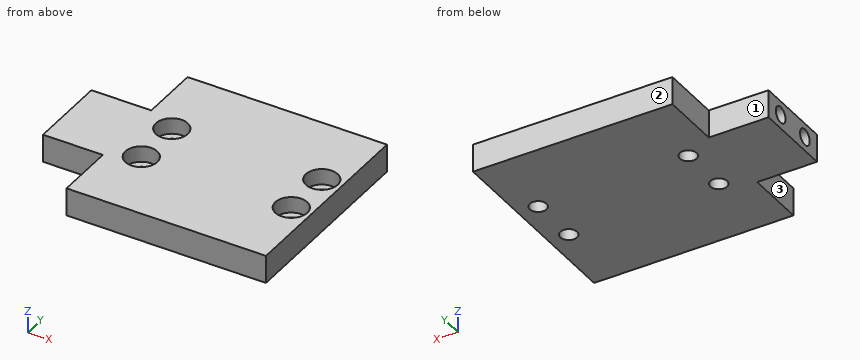
```python
from build123d import *

# Parameters (mm, degrees)
F1_DEPTH       = 7
F3_D           = 4
F3_DEPTH       = 6
F3_TIP         = 1.2017212381
F5_D           = 4.2
F5_CBORE_D     = 8
F5_CBORE_DEPTH = 4


with BuildPart() as f1:
    # F0 (on Top) → F1 (new body)
    with BuildSketch(Plane.XY):
        Polygon((32.5, -25), (32.5, 25), (-17.5, 25), (-17.5, 10), (-32.5, 10), (-32.5, -10), (-17.5, -10), (-17.5, -25), align=None)
    extrude(amount=F1_DEPTH)

    # F3
    with Locations(Plane(origin=(-32.5, 0, 0), x_dir=(0, -1, 0), z_dir=(-1, 0, 0))):
        with Locations((-5, 3.5), (5, 3.5)):
            Hole(F3_D / 2, depth=F3_DEPTH)
            with Locations((0, 0, -(F3_DEPTH + F3_TIP / 2))):  # 118° drill point
                Cone(0, F3_D / 2, F3_TIP, mode=Mode.SUBTRACT)

    # F5 (through all)
    with Locations(Plane.XY.offset(7)):
        with Locations((-10.1, 6.3), (-10.1, -6.3), (27.5, -6.3), (27.5, 6.3)):
            CounterBoreHole(F5_D / 2, F5_CBORE_D / 2, F5_CBORE_DEPTH)


solid = f1.part
```
Check sheet for the modelled part. Datum: model origin and axes. Units: mm. Face numbers are marked on the shaded views. A direction names the side the tool comes from. Round coordinates to 2 decimals unless told otherwise and drop trailing zeros. Write each loop counter-clockwise with the first axis right and the second up, starting at its lowest first coordinate (ties: lowest second). Pieces come first, ordered by that corner, then holes. Notation, with made-up numbers: M 0,-28.5 L 44,-28.5 A25 ccw 44,-1.5 Z; hole C -5.5,3.5 d10. An arc over 180 degrees is marked long. Write item = value, one per line. Start each with the question number.
1. Tool access check on the marked faces 1, 2 and 3. Record the directions out of +Z, -Z, +X, -X, +Y, -Y that give a thin tool (end or side, any length) a straight path to the whole face; none if there is none.
2. Scan lines: line 1 (Y direction, x = 27.5, z = 4.75); line 2 (X direction, y = 9, z = 4.25); line 3 (Y direction, x = -8, z = 3.5). Record each from-to range of solid material in increasing order. Write a range as [from, to].
3. Section check A-A, the plane x = 27.5. Record the cut outline in (y, z).
4. Section check D-D, the plane y = 6.3. State how many separate pieces and enclosed holes the cut face has, then the cut area to 3 significant figures.
5. Gauge pin test, flat ends, axial feed: pin 1 (2 mm diameter, centred on x = -18, y = 6, fed in from -Z); pin 2 (2 mm diameter, centred on y = 14.5, z = 4, fed in from -X); pin 3 (4 mm diameter, centred on x = 26.5, y = 7.5, fed in from +Z); pin 4 (3 mm diameter, centred on y = 5, z = 3.5, fed in from -X). Record the tip position at first contact, or that the pin passes through.
6. Section check C-C, the plane x = -11.5. Record the cut outline in (y, z), then the cut area to 3 significant figures.
7. Section check B-B, the plane y = -15. Record the cut outline in (x, z).
Results found:
q1.face_1 = +Z, -Z, -X, +Y
q1.face_2 = +Z, -Z, +X, -X, +Y
q1.face_3 = +Z, -Z, -X, -Y
q2.line_1 = [-25, -10.3], [-2.3, 2.3], [10.3, 25]
q2.line_2 = [-32.5, -13.05], [-7.15, 24.55], [30.45, 32.5]
q2.line_3 = [-25, -9.7], [-2.9, 2.9], [9.7, 25]
q3.outline = M -25,0 L -8.4,0 L -8.4,3 L -10.3,3 L -10.3,7 L -25,7 Z; M -4.2,0 L 4.2,0 L 4.2,3 L 2.3,3 L 2.3,7 L -2.3,7 L -2.3,3 L -4.2,3 Z; M 8.4,0 L 25,0 L 25,7 L 10.3,7 L 10.3,3 L 8.4,3 Z
q4.separate_pieces = 3
q4.enclosed_holes = 0
q4.area = 347 mm^2
q5.pin_1 = 0
q5.pin_2 = -17.5
q5.pin_3 = 3
q5.pin_4 = -26.2
q6.outline = M -25,0 L -7.87,0 L -7.87,3 L -10.05,3 L -10.05,7 L -25,7 Z; M -4.73,0 L 4.73,0 L 4.73,3 L 2.55,3 L 2.55,7 L -2.55,7 L -2.55,3 L -4.73,3 Z; M 7.87,0 L 25,0 L 25,7 L 10.05,7 L 10.05,3 L 7.87,3 Z
q6.area = 271 mm^2
q7.outline = M -17.5,0 L 32.5,0 L 32.5,7 L -17.5,7 Z
